CAD build for the part. Positions are in the model's coordinates, mm. Face numbers are marked on the shaded views. A direction names the side the tool comes from. Round coordinates to 2 decimals unless told otherwise and drop trailing zeros. Write each loop counter-clockwise with the first axis right and the second up, starting at its lowest first coordinate (ties: lowest second). Pieces come first, ordered by that corner, then holes. Notation, with made-up numbers: (24, -40) -> (47, -40) arc R20 ccw to (47, -3) -> close; hole circle Ø2 at (72.5, 78). An arc over 180 degrees is marked (long way). Answer in a Markdown table with one row per item. Add a question column.
```python
from build123d import *

# Parameters (mm, degrees)
F0_W     = 73
F0_H     = 82
F0_W_2   = 20.5
F0_H_2   = 15.5
F0_W_3   = 18
F0_H_3   = 43
F1_DEPTH = 3
F2_DEPTH = 20
F3_DEPTH = 15


with BuildPart() as f1:
    # F0 (on Top) → F1 (new body)
    with BuildSketch(Plane.XY):
        Rectangle(F0_W, F0_H)
        with Locations((-10.25, -23.95)):
            Rectangle(F0_W_2, F0_H_2, mode=Mode.SUBTRACT)
        with Locations((-10.25, -2.45)):
            Rectangle(F0_W_2, F0_H_2, mode=Mode.SUBTRACT)
        with Locations((17, -2.5)):
            Rectangle(F0_W_3, F0_H_3, mode=Mode.SUBTRACT)
        with Locations((-10.25, 19.05)):
            Rectangle(F0_W_2, F0_H_2, mode=Mode.SUBTRACT)
        with Locations((17, -2.5)):
            Rectangle(F0_W_3, F0_H_3)
        with Locations((-10.25, -2.45)):
            Rectangle(F0_W_2, F0_H_2)
        with Locations((-10.25, -23.95)):
            Rectangle(F0_W_2, F0_H_2)
        with Locations((-10.25, 19.05)):
            Rectangle(F0_W_2, F0_H_2)
    extrude(amount=-F1_DEPTH)

    # F0 (on Top) → F2 (join)
    with BuildSketch(Plane.XY):
        with Locations((-10.25, -23.95)):
            Rectangle(F0_W_2, F0_H_2)
        with Locations((-10.25, -2.45)):
            Rectangle(F0_W_2, F0_H_2)
        with Locations((-10.25, 19.05)):
            Rectangle(F0_W_2, F0_H_2)
    extrude(amount=F2_DEPTH)

    # F0 (on Top) → F3 (join)
    with BuildSketch(Plane.XY):
        with Locations((17, -2.5)):
            Rectangle(F0_W_3, F0_H_3)
    extrude(amount=F3_DEPTH)


solid = f1.part
```
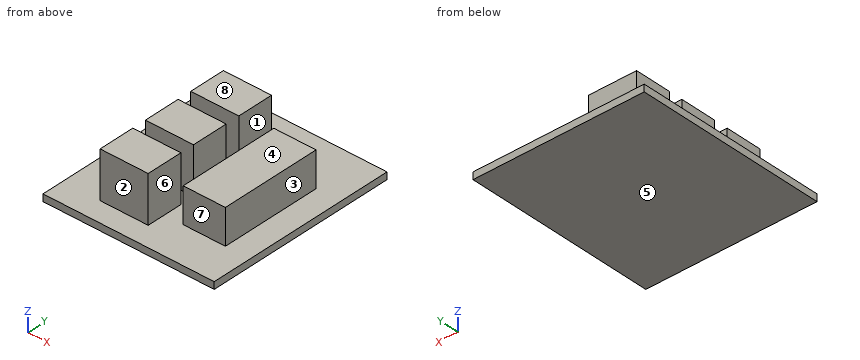
Item 1: Saw through at B-B on y = 21. Give the cut face in (x, z).
Item 2: Pin check, flat tips, straight feed: pin 1 (1 mm diameter, centred on x = -22, z = 13.5, fed in from +Y); pin 2 (6 mm diameter, centred on x = -13, z = 7.5, fed in from -Y); pin 3 (10 mm diameter, centred on x = -14.5, z = 13.5, fed in from +Y); pin 4 (8 mm diameter, centred on y = 0, z = 13.5, fed in from -X). Stop position of each tip, or through.
Item 3: Saw through at C-C on x = 23. Give the cut face in (y, z), then the cut area to 3 significant figures.
Item 4: Saw through at D-D on z = 18. Give the cut face in (x, y), then the cut area to 3 significant figures.
Item 5: Drill centre lines: probe 1 along Y at (x, z) = (-4, 13); probe 2 along X at (y, z) = (17.5, 5.75); probe 3 along Z at (x, y) = (6, -15). Where is each one in solid material? Low to high.
Item 6: Two-plate mould, pull along X, no slides. Class the marked faces 1, 2 and 3: +X half, -X half, draft (parallel to the pull), parting line (faces both ways), or undercut.
Item 7: Tool access for the marked faces 4, 5, 6, 7 and 8: list every direction of +Z, -Z, +X, -X, +Y, -Y with a clear straight run to the whole face (end or side of a thin tool).
Item 8: Saw through at A-A on z = 4.25. Give the cut face in (x, y), then the cut area to 3 significant figures.
Recorded:
| question | item | result |
|---|---|---|
| 1 | outline | (-36.5, -3) -> (36.5, -3) -> (36.5, 0) -> (0, 0) -> (0, 20) -> (-20.5, 20) -> (-20.5, 0) -> (-36.5, 0) -> close |
| 2 | pin 1 | through |
| 2 | pin 2 | y = -31.7 |
| 2 | pin 3 | y = 26.8 |
| 2 | pin 4 | x = -20.5 |
| 3 | outline | (-41, -3) -> (41, -3) -> (41, 0) -> (19, 0) -> (19, 15) -> (-24, 15) -> (-24, 0) -> (-41, 0) -> close |
| 3 | area | 891 mm2 |
| 4 | outline | (-20.5, -31.7) -> (0, -31.7) -> (0, -16.2) -> (-20.5, -16.2) -> close; (-20.5, -10.2) -> (0, -10.2) -> (0, 5.3) -> (-20.5, 5.3) -> close; (-20.5, 11.3) -> (0, 11.3) -> (0, 26.8) -> (-20.5, 26.8) -> close |
| 4 | area | 953 mm2 |
| 5 | probe 1 | -31.7 to -16.2, -10.2 to 5.3, 11.3 to 26.8 |
| 5 | probe 2 | -20.5 to 0, 8 to 26 |
| 5 | probe 3 | -3 to 0 |
| 6 | face 1 | undercut |
| 6 | face 2 | draft |
| 6 | face 3 | +X half |
| 7 | face 4 | +Z, +X, +Y, -Y |
| 7 | face 5 | -Z, +X, -X, +Y, -Y |
| 7 | face 6 | +Z, +Y, -Y |
| 7 | face 7 | +Z, +X, -Y |
| 7 | face 8 | +Z, +X, -X, +Y, -Y |
| 8 | outline | (-20.5, -31.7) -> (0, -31.7) -> (0, -16.2) -> (-20.5, -16.2) -> close; (-20.5, -10.2) -> (0, -10.2) -> (0, 5.3) -> (-20.5, 5.3) -> close; (-20.5, 11.3) -> (0, 11.3) -> (0, 26.8) -> (-20.5, 26.8) -> close; (8, -24) -> (26, -24) -> (26, 19) -> (8, 19) -> close |
| 8 | area | 1,730 mm2 |
